Can you work these out from the model? Positions are in its coordinate system, mm. Face numbers are marked on the shaded views. Coordinates: 2 decimals unless noted, no trailing zeros. Loops run counter-clockwise (first coordinate to the right, second up) from the corner with the lowest first, then second, coordinate; pieces in that order, holes last. Notation, with made-up numbers: M 24.25,79.5 L 59.25,79.5 A34 ccw 59.25,116.5 Z; hole C -2,85 d4. An arc over 180 degrees is marked long. Answer as a JSON object with one key per item and string values. Group by question number.
Item 1: I'm going to push flat-ended pins straight in: pin 1 Ø3 at (y, z) = (-4, 9) entering from +X; pin 2 Ø7.5 at (x, y) = (-12.7, 6.35) entering from +Z; pin 3 Ø2.5 at (x, y) = (12.7, -6.35) entering from -Z. Where does each tip first touch, or does it pass through?
Item 2: If I drill on line 1 (Y direction, x = -12.7, z = 4); line 2 (X direction, y = 7.5, z = 1.5); line 3 (X direction, y = -7, z = 10), over which ranges is the centre line in solid material (lowest first)?
Item 3: Suppose I cut it at B-B (z = 3.5). Write out the boundary of the cut face in (x, y).
Item 4: Suppose I cut it at C-C (y = 7). Count the separate pieces of the cut face and the enclosed holes in it, then the cut area to 3 significant figures.
Item 5: We'd pull the mould along Y, two halves only. Please class the marked faces 1, 2 and 3: +Y half, -Y half, draft (parallel to the pull), parting line (faces both ways), or undercut.
Item 6: Suppose I cut it at A-A (x = -12.7). Write out the boundary of the cut face in (y, z).
```python
from build123d import *

# Parameters (mm, degrees)
F1_DEPTH       = 12.7
F3_D           = 4.572
F3_CSINK_D     = 8.128
F3_CSINK_ANGLE = 90
F4_SIZE        = 1.27


with BuildPart() as f1:
    # F0 (on Top) → F1 (new body)
    with BuildSketch(Plane.XY):
        with BuildLine():
            Line((21.997045, 12.7), (-21.997045, 12.7))
            ThreePointArc((-21.997045, 12.7), (-25.4, 0), (-21.997045, -12.7))
            Line((-21.997045, -12.7), (21.997045, -12.7))
            ThreePointArc((21.997045, -12.7), (25.4, 0), (21.997045, 12.7))
        make_face()
    extrude(amount=F1_DEPTH)

    # F3 (through all)
    with Locations(Plane.XY.offset(12.7)):
        with Locations((-12.7, 6.35), (-12.7, -6.35), (12.7, -6.35), (12.7, 6.35)):
            CounterSinkHole(F3_D / 2, F3_CSINK_D / 2, counter_sink_angle=F3_CSINK_ANGLE)

    # F4
    f4_edges = [f1.edges().sort_by_distance(p)[0] for p in [
        (0, -12.7, 12.7),
        (25.4, 0, 12.7),
        (0, 12.7, 12.7),
        (-25.4, 0, 12.7),
    ]]
    chamfer(f4_edges, length=F4_SIZE)


solid = f1.part
```
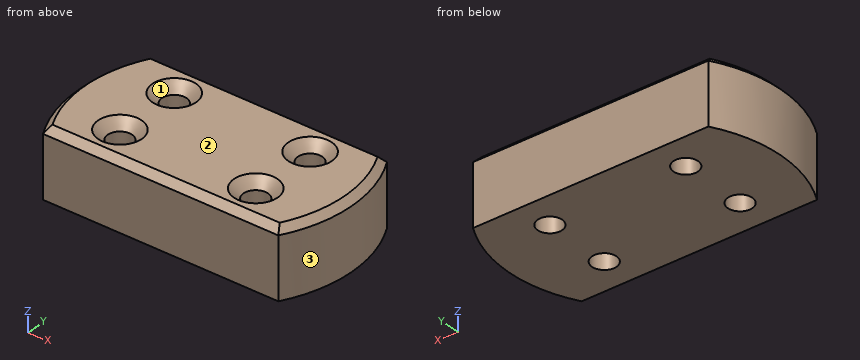
From the geometry:
{
 "1": {"pin 1": "x = 25.28", "pin 2": "z = 12.39", "pin 3": "through"},
 "2": {"line 1": "-12.7 to -8.64, -4.06 to 4.06, 8.64 to 12.7", "line 2": "-24.27 to -14.68, -10.72 to 10.72, 14.68 to 24.27", "line 3": "-24.42 to -14.89, -10.51 to 10.51, 14.89 to 24.42"},
 "3": {"outline": "M -22,-12.7 L 22,-12.7 A25.4 ccw 22,12.7 L -22,12.7 A25.4 ccw Z; hole C -12.7,-6.35 d4.57; hole C -12.7,6.35 d4.57; hole C 12.7,-6.35 d4.57; hole C 12.7,6.35 d4.57"},
 "4": {"separate pieces": "3", "enclosed holes": "0", "area": "501 mm2"},
 "5": {"face 1": "undercut", "face 2": "draft", "face 3": "parting line"},
 "6": {"outline": "M -12.7,0 L -8.64,0 L -8.64,10.92 L -10.41,12.7 L -11.43,12.7 L -12.7,11.43 Z; M -4.06,0 L 4.06,0 L 4.06,10.92 L 2.29,12.7 L -2.29,12.7 L -4.06,10.92 Z; M 8.64,0 L 12.7,0 L 12.7,11.43 L 11.43,12.7 L 10.41,12.7 L 8.64,10.92 Z"}
}
